Build history of the part. All positions in model axes, mm. Face numbers are marked on the shaded views. A direction names the side the tool comes from. Coordinates: 2 decimals unless noted, no trailing zeros. Loops run counter-clockwise (first coordinate to the right, second up) from the corner with the lowest first, then second, coordinate; pieces in that order, holes last.
Item 1: Cut at A-A (y = -23). List the corners of the cut face in (x, z), and give its area (4 significant figures).
Item 2: 3-axis set-ups, long thin cutter, end or side, ignore diameter. For the marked faces 1 and 2: which of +Z, -Z, +X, -X, +Y, -Y reach the whole face in a straight line?
Item 3: Mould opens along Y. For the marked faces 3, 4, 5 and 6 say: released by +Y, released by -Y, zero draft, split by the parting line, or undercut.
Item 4: Flat gauge pins, fed straight in: pin 1 (1 mm diameter, centred on x = -3.5, y = 16.5, fed in from -Z); pin 2 (10 mm diameter, centred on x = -23.5, y = -6, fed in from +Z). Where does each tip first touch, or does it go through?
Item 5: Drill centre lines: line 1 along X through (y, z) = (-25, 27.5); line 2 along Y through (x, z) = (-3, 23.5); line 3 along Z through (x, y) = (-6, 19). Where is each one in solid material? Low to high.
Item 6: Cut at C-C (x = -31). List the corners of the cut face in (y, z).
Item 7: Cut at B-B (z = 16.5). List the corners of the cut face in (x, y).
from build123d import *

# Parameters (mm, degrees)
F0_W     = 74
F0_H     = 57
F1_DEPTH = 40
F2_R     = 2.5
F3_W     = 71
F3_H     = 54
F4_DEPTH = 25
F5_R     = 1.5


with BuildPart() as f1:
    # F0 (on Top) → F1 (new body)
    with BuildSketch(Plane.XY):
        Rectangle(F0_W, F0_H)
    extrude(amount=F1_DEPTH)

    # F2
    f2_edges = [f1.edges().sort_by_distance(p)[0] for p in [
        (37, 28.5, 20),
        (37, -28.5, 20),
        (-37, -28.5, 20),
        (-37, 28.5, 20),
    ]]
    fillet(f2_edges, radius=F2_R)

    # F3 (on face) → F4 (cut)
    with BuildSketch(Plane.XY.offset(40)):
        Rectangle(F3_W, F3_H)
    extrude(amount=-F4_DEPTH, mode=Mode.SUBTRACT)

    # F5
    f5_edges = [f1.edges().sort_by_distance(p)[0] for p in [
        (35.5, -27, 27.5),
        (-35.5, -27, 27.5),
        (-35.5, 27, 27.5),
        (35.5, 27, 27.5),
    ]]
    fillet(f5_edges, radius=F5_R)


solid = f1.part
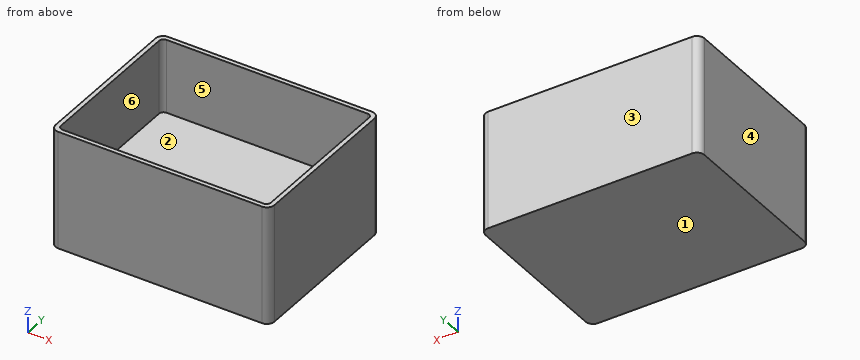
Filled sheet:
1. outline: (-37, 0) - (37, 0) - (37, 40) - (35.5, 40) - (35.5, 15) - (-35.5, 15) - (-35.5, 40) - (-37, 40) - close
1. area: 1,185 mm2
2. face 1: -Z, +X, -X, +Y, -Y
2. face 2: +Z
3. face 3: released by +Y
3. face 4: zero draft
3. face 5: undercut
3. face 6: undercut
4. pin 1: stops at z = 0
4. pin 2: stops at z = 15
5. line 1: x = -37 to -35.5, 35.5 to 37
5. line 2: y = -28.5 to -27, 27 to 28.5
5. line 3: z = 0 to 15
6. outline: (-28.5, 0) - (28.5, 0) - (28.5, 40) - (27, 40) - (27, 15) - (-27, 15) - (-27, 40) - (-28.5, 40) - close
7. outline: (-37, -26) arc R2.5 ccw to (-34.5, -28.5) - (34.5, -28.5) arc R2.5 ccw to (37, -26) - (37, 26) arc R2.5 ccw to (34.5, 28.5) - (-34.5, 28.5) arc R2.5 ccw to (-37, 26) - close; hole (-35.5, -25.5) arc R1.5 ccw to (-34, -27) - (34, -27) arc R1.5 ccw to (35.5, -25.5) - (35.5, 25.5) arc R1.5 ccw to (34, 27) - (-34, 27) arc R1.5 ccw to (-35.5, 25.5) - close
